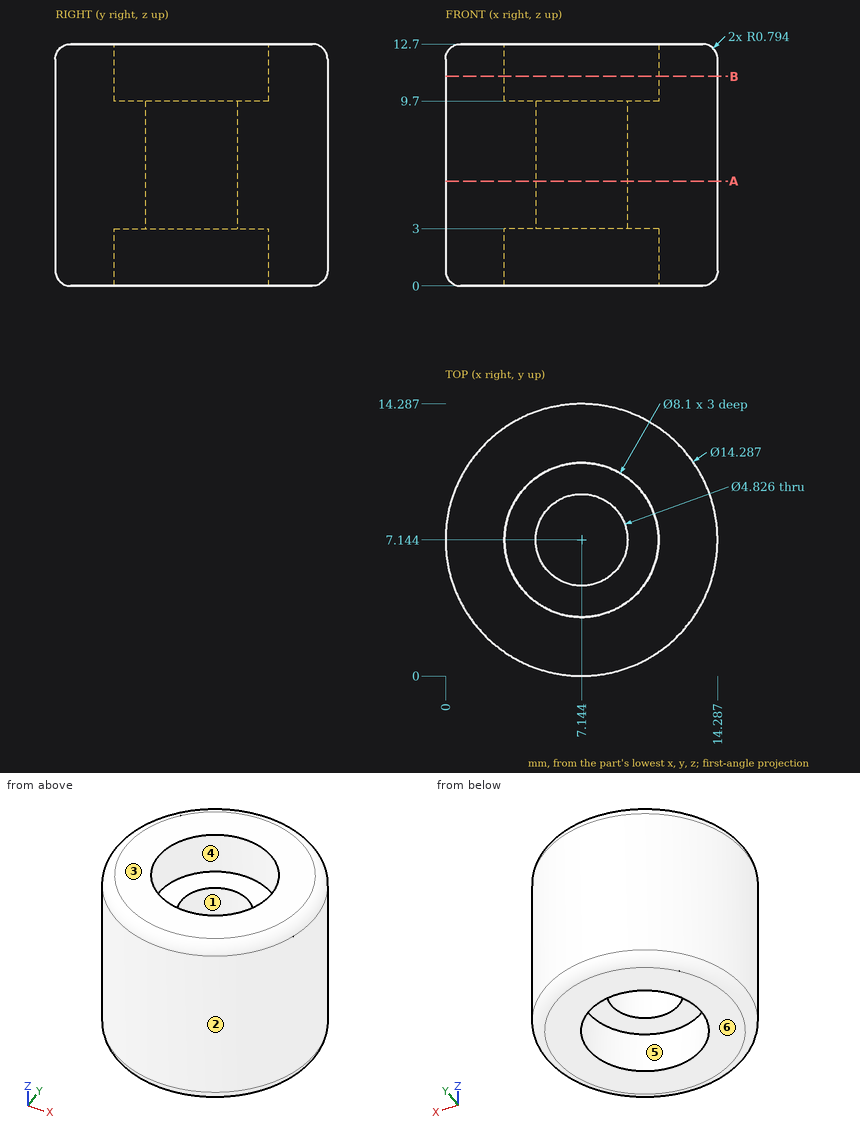
Study the drawing (mm; zero at the part's minimum x, y, z) and answer. A direction names the side the tool comes from. Give positions to 0.01 mm unless a question says otherwise; leave off trailing zeros. Loops run counter-clockwise (first coordinate to the right, second up) from the corner with the lowest first, then second, coordinate; pieces in that order, holes last. Notation, with made-up numbers: (16, -17.75) - (50, -17.75) arc R25 ccw to (50, 1.25) - close; hole circle Ø9 at (51.5, 33). An arc over 180 degrees is marked (long way). Return JSON: item names as keys, results as strings. Group by question number.
1. Determine the mould class of the marked faces 1, 2 and 3 for opening direction Y: pulls with the +Y half, pulls with the -Y half, needs draft (parallel to the pull), parting line crosses it, or undercut.
2. Find section A-A (z = 5.5). Write down the section's boundary in (x, y) (1 decimal).
3. Given pin 1 Ø5.5 at (x, y) = (7.14, 7.14) entering from -Z; pin 2 Ø5 at (y, z) = (2.5, 7) entering from -X; pin 3 Ø2 at (y, z) = (11, 6) entering from +X, each flat-ended and moving along its own axis, determine where each tip first touches the part or whether it passes through.
4. Which of the six approach directions +Z, -Z, +X, -X, +Y, -Y give full straight-line access (tool end or side, diameter ignored) to the marked faces 4, 5 and 6?
5. Find section B-B (z = 11). Write down the section's boundary in (x, y), then the cut area to 3 significant figures.
6. Straight lines are drawn through the part: line 1 (X direction, y = 7, z = 2) (1 decimal); line 2 (Y direction, x = 6, z = 6.75) (1 decimal). For each, find the intervals that lie inside material, in ascending order. Write a range as [from, to].
Verdict:
{
 "1": {"face 1": "undercut", "face 2": "parting line crosses it", "face 3": "needs draft"},
 "2": {"outline": "circle Ø14.3 at (7.1, 7.1); hole circle Ø4.8 at (7.1, 7.1)"},
 "3": {"pin 1": "stops at z = 3", "pin 2": "stops at x = 0.33", "pin 3": "stops at x = 13.69"},
 "4": {"face 4": "+Z", "face 5": "-Z", "face 6": "-Z, +X, -X, +Y, -Y"},
 "5": {"outline": "circle Ø14.29 at (7.14, 7.14); hole circle Ø8.1 at (7.14, 7.14)", "area": "109 mm^2"},
 "6": {"line 1": "x = [0, 3.1], [11.2, 14.3]", "line 2": "y = [0.1, 5], [9.3, 14.2]"}
}
